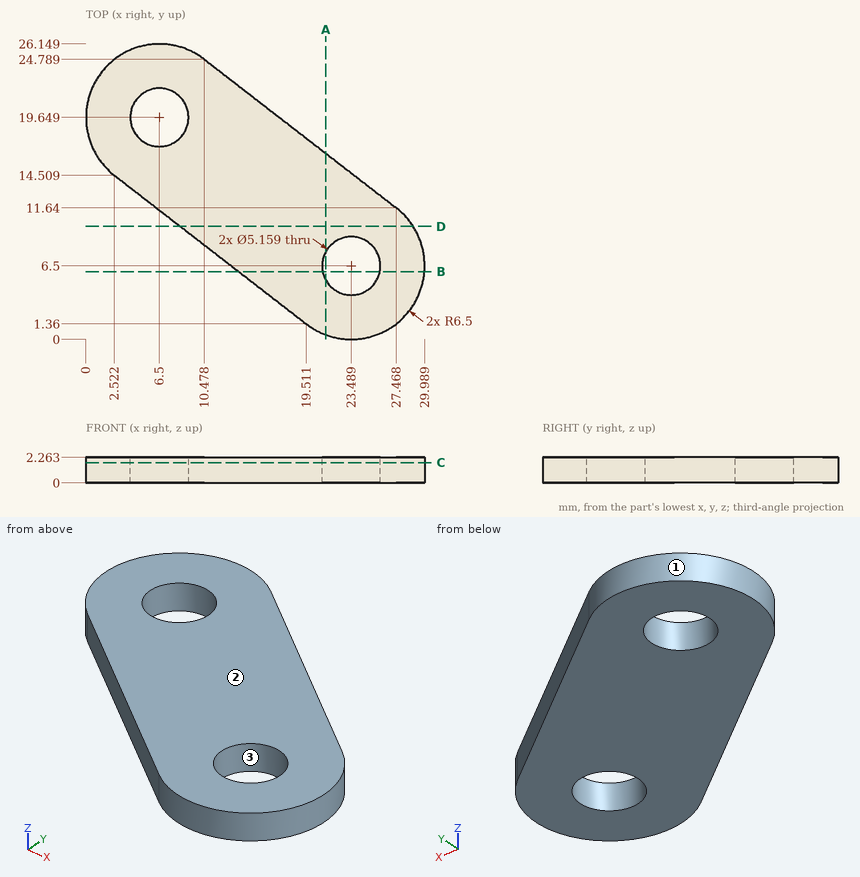
Here's the drawing with two shaded views (mm, measured from the low corner). I have some questions. Round coordinates to 2 decimals unless told otherwise and drop trailing zeros. Write each loop counter-clockwise with the first axis right and the second up, starting at its lowest first coordinate (ties: lowest second). Pieces come first, ordered by that corner, then holes. Notation, with made-up numbers: M -35.75,-36.5 L 0.25,-36.5 A28 cw 0.25,-2.5 Z; hole C 55.5,42.25 d3. An arc over 180 degrees is marked long. Answer in a Markdown table with one row per item. Add a question column.
Q1. Imagine slicing it at D-D (y = 10). Please give me the cut outline in (x, z).
Q2. Imagine slicing it at B-B (y = 6). Please give me the cut outline in (x, z) (1 decimal).
Q3. Imagine slicing it at A-A (x = 21.25). Please give me the cut outline in (y, z).
Q4. Imagine slicing it at C-C (z = 1.8). Please give me the cut outline in (x, y), then the cut area to 3 significant figures.
Q5. Will this pin go through, and if not, where does the flat tip stop? pin 1 Ø1 at (x, z) = (18, 0.5) entering from +Y (1 decimal).
Q6. If we mould it in two halves opening along Y, with no side actions, what happens to the marked faces 1, 2 and 3? For each: +Y half, -Y half, draft (parallel to the pull), parting line (faces both ways), or undercut.
Q7. If I drill on line 1 (X direction, y = 17.5, z = 0.3) (1 decimal); line 2 (Y direction, x = 5.25, z = 1.4) (1 decimal); line 3 (X direction, y = 19, z = 1.65) (1 decimal), over which ranges is the centre line in solid material (lowest first)? Write a range as from..to.
Values:
| question | item | result |
|---|---|---|
| 1 | outline | M 8.35,0 L 28.97,0 L 28.97,2.26 L 8.35,2.26 Z |
| 2 | outline | M 13.5,0 L 21,0 L 21,2.3 L 13.5,2.3 Z; M 26,0 L 30,0 L 30,2.3 L 26,2.3 Z |
| 3 | outline | M 0.4,0 L 5.22,0 L 5.22,2.26 L 0.4,2.26 Z; M 7.78,0 L 16.45,0 L 16.45,2.26 L 7.78,2.26 Z |
| 4 | outline | M 2.52,14.51 L 19.51,1.36 A6.5 ccw 27.47,11.64 L 10.48,24.79 A6.5 ccw Z; hole C 6.5,19.65 d5.16; hole C 23.49,6.5 d5.16 |
| 4 | area | 370 mm^2 |
| 5 | pin 1 | y = 19.4 |
| 6 | face 1 | parting line |
| 6 | face 2 | draft |
| 6 | face 3 | undercut |
| 7 | line 1 | 0.4..5.1, 7.9..19.9 |
| 7 | line 2 | 12.4..17.4, 21.9..26 |
| 7 | line 3 | 0..4, 9..18 |
